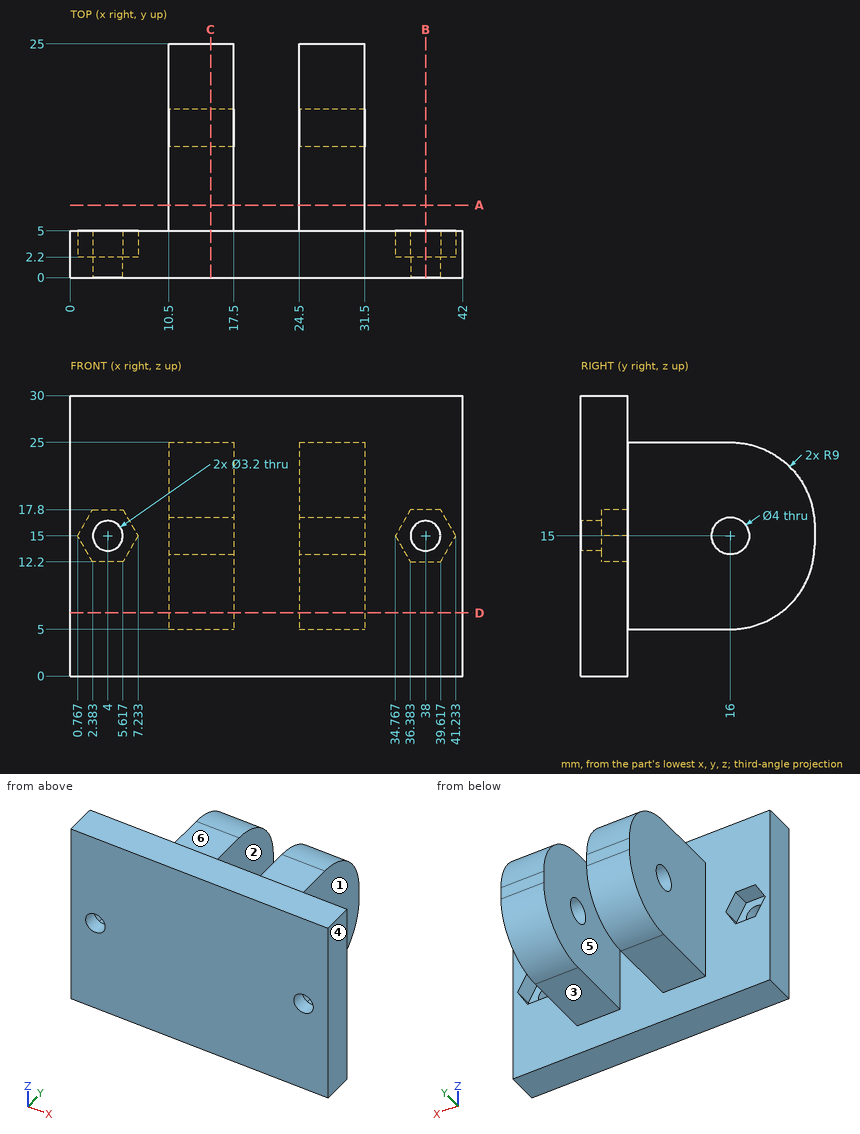
Answer from the drawing. Dimensions are ordinates in mm from the lowest x, y and z of the part. A direction names the side the tool comes from. Coordinates: 2 decimals unless noted, no trailing zeros. Order: outer loops, then holes, each group sorted by start corner. A loop starts at its lowest first (then second) coordinate and runs counter-clockwise, first axis right, second up. Notation, with made-up numbers: M 7,22 L 40,22 A24 ccw 40,39 Z; hole C 89.5,53 d3. An arc over 180 degrees is marked long. Put each result on its own line as item: value. Start each with the question number.
Item 1: Section D-D, the plane z = 6.75 is taken. Determine the outline of the cut face in (x, y).
Item 2: Section A-A, the plane y = 7.75 is taken. Determine the outline of the cut face in (x, z), plus the area to 3 significant figures.
Item 3: The mould has two halves that part along X. Classify the marked faces 4, 5 and 6: +X half, -X half, draft (parallel to the pull), parting line (faces both ways), or undercut.
Item 4: Section C-C, the plane x = 15 is taken. Determine the outline of the cut face in (y, z).
Item 5: Consider probe 1 along X at (y, z) = (16.5, 12); probe 2 along Y at (x, z) = (14, 15); probe 3 along Y at (x, z) = (9.5, 22). Determine where each line is inside the solid, lowest interval first. Write a range as [from, to].
Item 6: Given pin 1 Ø5 at (y, z) = (11, 11) entering from +X; pin 2 Ø8 at (x, y) = (23, 12.5) entering from +Z; pin 3 Ø3.5 at (x, y) = (13.5, 9.5) entering from -Z, each flat-ended and moving along its own axis, determine where each tip first touches the part or whether it passes through.
Item 7: For the marked faces 1, 2 and 3, determine the directions among +Z, -Z, +X, -X, +Y, -Y from which every point of the face is accessible in a straight line to the end or side of a thin tool.
Item 8: Section B-B, the plane x = 38 is taken. Determine the outline of the cut face in (y, z).
Computed:
1. outline: M 0,0 L 42,0 L 42,5 L 31.5,5 L 31.5,21.33 L 24.5,21.33 L 24.5,5 L 17.5,5 L 17.5,21.33 L 10.5,21.33 L 10.5,5 L 0,5 Z
2. outline: M 10.5,5 L 17.5,5 L 17.5,25 L 10.5,25 Z; M 24.5,5 L 31.5,5 L 31.5,25 L 24.5,25 Z
2. area: 280 mm2
3. face 4: +X half
3. face 5: undercut
3. face 6: draft
4. outline: M 0,0 L 5,0 L 5,5 L 16,5 A9 ccw 25,14 L 25,16 A9 ccw 16,25 L 5,25 L 5,30 L 0,30 Z; hole C 16,15 d4
5. probe 1: x = [10.5, 17.5], [24.5, 31.5]
5. probe 2: y = [0, 14], [18, 25]
5. probe 3: y = [0, 5]
6. pin 1: stops at x = 31.5
6. pin 2: stops at z = 25
6. pin 3: stops at z = 5
7. face 1: +Z, -Z, +X, +Y
7. face 2: +Z, -Z, +Y
7. face 3: -Z, +X, -X, +Y
8. outline: M 0,0 L 5,0 L 5,12.2 L 2.2,12.2 L 2.2,13.4 L 0,13.4 Z; M 0,16.6 L 2.2,16.6 L 2.2,17.8 L 5,17.8 L 5,30 L 0,30 Z
